Read the model definition and answer for the solid it produces. Units are mm, in the model's axes. A direction names the side the tool comes from. Coordinates: 2 decimals unless noted, no trailing zeros. Write each loop counter-clockwise with the first axis right and the second up, starting at its lowest first coordinate (ties: lowest second). Pieces come first, ordered by that corner, then holes. Notation, with made-up numbers: (44.5, -22.5) -> (95.5, -22.5) arc R28 cw to (95.5, 0.5) -> close; hole circle Ø4 at (-4, 50.5). An arc over 180 degrees is marked (long way). One line per item, written item: value. Start each with the question number.
1. For faces 4 (the flat face through (0, -24, 7)), 5 (the flat face through (-30, 5, 5)), determine the directions among +Z, -Z, +X, -X, +Y, -Y from which every point of the face is accessible in a straight line to the end or side of a thin tool.
2. Find section C-C, the plane y = 29.5. Write down the section's boundary in (x, z).
3. Find section B-B, the plane z = 10. Write down the section's boundary in (x, y).
4. Find section A-A, the plane y = 0. Write down the section's boundary in (x, z), and give its area (3 significant figures).
5. Consider line 1 along Y through (x, z) = (0, 4); line 2 along Y through (x, z) = (0, 8); line 3 along X through (y, z) = (0, 7.85). Determine where each line is inside the solid, lowest interval first.
6. Given P1, Ø8, axis at x = 2, y = -11, coming from the +Z side; P2, Ø1.8, axis at x = -1, y = 22, coming from the +Z side; P3, Ø6, axis at x = -5.5, y = 19, coming from the +Z side, each flat-ended and moving along its own axis, determine where each tip first touches the part or whether it passes through.
7. Find section D-D, the plane x = -23. Write down the section's boundary in (y, z).
8. For a pull along Y with two mould halves and no side action, classify faces 1 (the cylindrical face through (8.767, -16.856, 7.592)), 2 (the flat face through (0, -25, 5)), 3 (the flat face through (0, 35, 5)) as pulls with the +Y half, pulls with the -Y half, needs draft (parallel to the pull), parting line crosses it, or undercut.
```python
from build123d import *

# Parameters (mm, degrees)
SKETCH_R             = 20
PAD_DEPTH            = 7
SKETCH001_R          = 3
PAD001_DEPTH         = 5
SKETCH002_R          = 20
SKETCH002_R_2        = 19
PAD002_DEPTH         = 8.2
SKETCH003_W          = 60
SKETCH003_H          = 60
PAD003_DEPTH         = 5
SKETCH004_W          = 60
SKETCH004_H          = 60
SKETCH004_W_2        = 58
SKETCH004_H_2        = 58
PAD004_DEPTH         = 15
SKETCH006_R          = 3
POCKET_DEPTH         = 4
SKETCH005_R          = 5
POCKET001_DEPTH      = 5.001
POCKET001_DEPTH_BACK = -15.001


with BuildPart() as part:
    # Sketch → Pad (new body)
    with BuildSketch(Plane.XY):
        Circle(SKETCH_R)
    extrude(amount=PAD_DEPTH)

    # Sketch001 → Pad001 (join)
    with BuildSketch(Plane.XY):
        with BuildLine():
            add(Edge.make_bspline(
                [(-12.484701, 15.624732), (-10.829835, 23.483566), (0, 31.619604), (10.829835, 23.483566), (12.484701, 15.624732)],
                knots=[0, 0, 0, 0, 0.5, 1, 1, 1, 1], degree=3))
            Line((12.484701, 15.624732), (-12.484701, 15.624732))
        make_face()
        with Locations((0, 23.512977)):
            Circle(SKETCH001_R, mode=Mode.SUBTRACT)
    extrude(amount=PAD001_DEPTH)

    # Sketch002 → Pad002 (join)
    with BuildSketch(Plane.XY):
        Circle(SKETCH002_R)
        Circle(SKETCH002_R_2, mode=Mode.SUBTRACT)
    extrude(amount=PAD002_DEPTH)

    # Sketch003 → Pad003 (join)
    with BuildSketch(Plane.XY):
        with Locations((0, 5)):
            Rectangle(SKETCH003_W, SKETCH003_H)
    extrude(amount=-PAD003_DEPTH)

    # Sketch004 → Pad004 (join)
    with BuildSketch(Plane.XY):
        with Locations((0, 5)):
            Rectangle(SKETCH004_W, SKETCH004_H)
        with Locations((0, 5)):
            Rectangle(SKETCH004_W_2, SKETCH004_H_2, mode=Mode.SUBTRACT)
    extrude(amount=PAD004_DEPTH)

    # Sketch006 → Pocket (cut)
    with BuildSketch(Plane.XY):
        with Locations((0, 23.512977)):
            Circle(SKETCH006_R)
    extrude(amount=-POCKET_DEPTH, mode=Mode.SUBTRACT)

    # Sketch005 → Pocket001 (cut, two sides)
    with BuildSketch(Plane.XY) as pocket001_sk:
        Circle(SKETCH005_R)
    extrude(amount=-POCKET001_DEPTH, mode=Mode.SUBTRACT)
    extrude(pocket001_sk.sketch, amount=-POCKET001_DEPTH_BACK, mode=Mode.SUBTRACT)


solid = part.part
```
Answer block:
1. face 4: +Z
1. face 5: +Z, -Z, -X, +Y, -Y
2. outline: (-30, -5) -> (30, -5) -> (30, 15) -> (29, 15) -> (29, 0) -> (-29, 0) -> (-29, 15) -> (-30, 15) -> close
3. outline: (-30, -25) -> (30, -25) -> (30, 35) -> (-30, 35) -> close; hole (-29, -24) -> (29, -24) -> (29, 34) -> (-29, 34) -> close
4. outline: (-30, -5) -> (-5, -5) -> (-5, 7) -> (-19, 7) -> (-19, 8.2) -> (-20, 8.2) -> (-20, 0) -> (-29, 0) -> (-29, 15) -> (-30, 15) -> close; (5, -5) -> (30, -5) -> (30, 15) -> (29, 15) -> (29, 0) -> (20, 0) -> (20, 8.2) -> (19, 8.2) -> (19, 7) -> (5, 7) -> close
4. area: 492 mm2
5. line 1: y = -25 to -24, -20 to -5, 5 to 20.51, 26.51 to 27.55, 34 to 35
5. line 2: y = -25 to -24, -20 to -19, 19 to 20, 34 to 35
5. line 3: x = -30 to -29, -20 to -19, 19 to 20, 29 to 30
6. P1: stops at z = 7
6. P2: stops at z = -4
6. P3: stops at z = 8.2
7. outline: (-25, -5) -> (35, -5) -> (35, 15) -> (34, 15) -> (34, 0) -> (-24, 0) -> (-24, 15) -> (-25, 15) -> close
8. face 1: undercut
8. face 2: pulls with the -Y half
8. face 3: pulls with the +Y half
